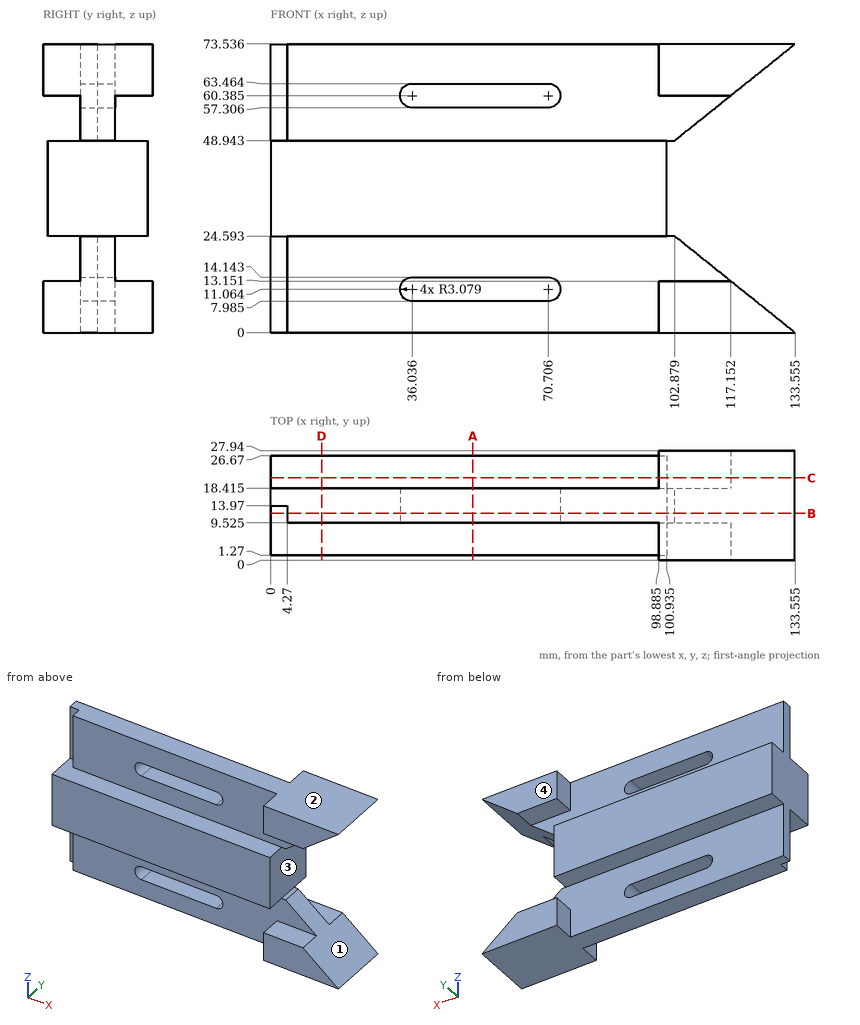
Could you check a few things on this drawing? It's one solid part, dimensions in mm from its lowest x, y, z. Round coordinates to 2 decimals unless told otherwise and drop trailing zeros. Order: outer loops, then holes, each group sorted by start corner. A loop starts at its lowest first (then second) coordinate and runs counter-clockwise, first axis right, second up.
(1) Imagine slicing it at A-A (x = 51.5). Write out the boundary of the cut face in (y, z) (1 decimal), plus the area to 3 significant figures.
Response values:
outline: (1.3, 24.6) - (9.5, 24.6) - (9.5, 14.1) - (18.4, 14.1) - (18.4, 24.6) - (26.7, 24.6) - (26.7, 48.9) - (18.4, 48.9) - (18.4, 57.3) - (9.5, 57.3) - (9.5, 48.9) - (1.3, 48.9) - close; (9.5, 0) - (18.4, 0) - (18.4, 8) - (9.5, 8) - close; (9.5, 63.5) - (18.4, 63.5) - (18.4, 73.5) - (9.5, 73.5) - close
area: 946 mm2
(2) Imagine slicing it at D-D (x = 13). Write out the boundary of the cut face in (y, z) (1 decimal), plus the area to 3 significant figures.
Response values:
outline: (1.3, 24.6) - (9.5, 24.6) - (9.5, 0) - (18.4, 0) - (18.4, 24.6) - (26.7, 24.6) - (26.7, 48.9) - (18.4, 48.9) - (18.4, 73.5) - (9.5, 73.5) - (9.5, 48.9) - (1.3, 48.9) - close
area: 1,060 mm2
(3) Please list where these lines run through material, in increasing order: line 1 along Z through (x, y) = (47, 10) (1 decimal); line 2 along Y through (x, z) = (76, 36.5); line 3 along X through (y, z) = (3, 34) (1 decimal).
Response values:
line 1: z = 0 to 8, 14.1 to 57.3, 63.5 to 73.5
line 2: y = 1.27 to 26.67
line 3: x = 0 to 100.9
(4) If we mould it in two halves opening along Z, with no side actions, what happens to the marked faces 1, 2, 3 and 4? For each: released by +Z, released by -Z, zero draft, split by the parting line, or undercut.
Response values:
face 1: undercut
face 2: released by +Z
face 3: undercut
face 4: zero draft
(5) I'm going to push flat-ended pins straight in: pin 1 (2 mm diameter, centred on y = 12.5, z = 16, fed in from -X); pin 2 (5 mm diameter, centred on y = 18, z = 11.5, fed in from +X); pin 3 (4 mm diameter, centred on x = 67.5, y = 7, fed in from -Z). Where does each tip first touch, or does it pass through?
Response values:
pin 1: stops at x = 4.27
pin 2: stops at x = 122.33
pin 3: stops at z = 24.59
(6) Imagine slicing it at B-B (y = 12). Write out the boundary of the cut face in (x, z) (1 decimal), plus the area to 3 significant figures.
Response values:
outline: (0, 24.6) - (4.3, 24.6) - (4.3, 0) - (133.6, 0) - (102.9, 24.6) - (100.9, 24.6) - (100.9, 48.9) - (102.9, 48.9) - (133.6, 73.5) - (4.3, 73.5) - (4.3, 48.9) - (0, 48.9) - close; hole (36, 8) - (70.7, 8) arc R3.1 ccw to (70.7, 14.1) - (36, 14.1) arc R3.1 ccw to start; hole (36, 57.3) - (70.7, 57.3) arc R3.1 ccw to (70.7, 63.5) - (36, 63.5) arc R3.1 ccw to start
area: 7,580 mm2
(7) Imagine slicing it at C-C (y = 21). Count the separate pieces of the cut face and the enclosed holes in it, plus the area to 3 significant figures.
Response values:
separate pieces: 3
enclosed holes: 0
area: 3,150 mm2
